```python
from build123d import *

# Parameters (mm, degrees)
SKETCH_1_R          = 1.7
EXTRUDE_1_DEPTH     = 2.5
SKETCH_3_R          = 3
SKETCH_3_R_2        = 1.7
EXTRUDE_2_DEPTH     = 4.3
EXTRUDE_3_DEPTH     = 2.5
EXTRUDE_4_DEPTH     = 2.5
CUT_EXTRUDE_2_DEPTH = 10
EXTRUDE_6_DEPTH     = 2.5
FILLET_START        = -1
FILLET_1_DEPTH      = 3.5
FILLET_1_2_DEPTH    = 2.5


with BuildPart() as part:
    # 草图1 → 凸台-拉伸1 (new body)
    with BuildSketch(Plane(origin=(0, 0, 0), x_dir=(1, 0, 0), z_dir=(0, 1, 0))):
        with BuildLine():
            Line((-10, 3), (10, 3))
            ThreePointArc((10, 3), (11.414213562, 2.414213562), (12, 1))
            Line((12, 1), (12, -1))
            ThreePointArc((12, -1), (11.414213562, -2.414213562), (10, -3))
            Line((10, -3), (-10, -3))
            ThreePointArc((-10, -3), (-11.414213562, -2.414213562), (-12, -1))
            Line((-12, -1), (-12, 1))
            ThreePointArc((-12, 1), (-11.414213562, 2.414213562), (-10, 3))
        make_face()
        with Locations(Location((-9, 0, 0), (0, 0, 270))):
            Circle(SKETCH_1_R, mode=Mode.SUBTRACT)
        with Locations(Location((9, 0, 0), (0, 0, 270))):
            Circle(SKETCH_1_R, mode=Mode.SUBTRACT)
    extrude(amount=EXTRUDE_1_DEPTH)

    # 草图3 → 凸台-拉伸2 (add)
    with BuildSketch(Plane(origin=(0, 2.5, 0), x_dir=(1, 0, 0), z_dir=(0, 1, 0))):
        with Locations(Location((-9, 0, 0), (0, 0, 270))):
            Circle(SKETCH_3_R)
        with Locations(Location((-9, 0, 0), (0, 0, 270))):
            Circle(SKETCH_3_R_2, mode=Mode.SUBTRACT)
    extrude(amount=EXTRUDE_2_DEPTH)

    # 草图4 → 凸台-拉伸3 (add)
    with BuildSketch(Plane.XZ):
        with BuildLine():
            Line((3, -3), (3, -6))
            add(Edge.make_bspline(
                [(9, -4), (5.683772234, -4.051316702), (3, -6)],
                knots=[0, 0, 0, 1, 1, 1], degree=2))
            add(Edge.make_bspline(
                [(9, -4), (12.316227766, -4.051316702), (15, -6)],
                knots=[0, 0, 0, 1, 1, 1], degree=2))
            Line((15, -6), (15, -3))
            Line((15, -3), (3, -3))
        make_face()
        with BuildLine():
            Line((3, 3), (15, 3))
            Line((15, 3), (15, 6))
            add(Edge.make_bspline(
                [(9, 4), (12.316227766, 4.051316702), (15, 6)],
                knots=[0, 0, 0, 1, 1, 1], degree=2))
            add(Edge.make_bspline(
                [(9, 4), (5.683772234, 4.051316702), (3, 6)],
                knots=[0, 0, 0, 1, 1, 1], degree=2))
            Line((3, 6), (3, 3))
        make_face()
    extrude(amount=-EXTRUDE_3_DEPTH)

    # 草图5 → 凸台-拉伸4 (add)
    with BuildSketch(Plane.XZ):
        Polygon((9.41538426, 3.145270203), (11.442509661, 0.357972777), (9.41538426, -3.078638254), (11.917617176, -3.601256521), (12, -3.235006375), (12, 3.620377719), align=None)
    extrude(amount=-EXTRUDE_4_DEPTH)

    # 草图10 → 切除-拉伸2 (cut)
    with BuildSketch(Plane.XZ):
        Polygon((9, 4), (14.708854471, 4.088341194), (15, 6), align=None)
        Polygon((9, -4), (14.512519064, -3.914696982), (15, -6), align=None)
    extrude(amount=-CUT_EXTRUDE_2_DEPTH, mode=Mode.SUBTRACT)

    # 草图11 → 凸台-拉伸6 (add)
    with BuildSketch(Plane.XZ):
        with BuildLine():
            Line((15, 6), (15, 3.4))
            Line((15, 3.4), (3, 3.4))
            Line((3, 3.4), (3, 8.6))
            add(Edge.make_bspline(
                [(3, 8.6), (3.743724888, 5.90317916), (8.383809549, 2.787162352), (13.287766409, 4.701526195), (15, 6)],
                knots=[0, 0, 0, 0, 0.541786912, 1, 1, 1, 1], degree=3))
        make_face()
        with BuildLine():
            Line((3, -8.6), (3, -3.580116595))
            Line((3, -3.580116595), (15, -3.580116595))
            Line((15, -3.580116595), (15, -6))
            add(Edge.make_bspline(
                [(15, -6), (13.28897523, -4.705122665), (8.381534555, -2.775849949), (3.754894418, -5.92427983), (3, -8.6)],
                knots=[0, 0, 0, 0, 0.458377401, 1, 1, 1, 1], degree=3))
        make_face()
    extrude(amount=-EXTRUDE_6_DEPTH)

    # 圆角1: read off the stored shape, not the designer's step
    # 圆角1 outline → 圆角1 (cut)
    with BuildSketch(Plane(origin=(0, 0, 0), x_dir=(1, 0, 0), z_dir=(0, 1, 0)).offset(FILLET_START)):
        with BuildLine():
            Line((15, -3), (13.5, -3))
            ThreePointArc((13.5, -3), (14.560660172, -3.439339828), (15, -4.5))
            Line((15, -4.5), (15, -3))
        make_face()
        with BuildLine():
            ThreePointArc((15, 4.5), (14.560660172, 3.439339828), (13.5, 3))
            Line((13.5, 3), (15, 3))
            Line((15, 3), (15, 4.5))
        make_face()
    extrude(amount=FILLET_1_DEPTH, mode=Mode.SUBTRACT)

    # Fillet 1 2 outline → Fillet 1 2 (add)
    with BuildSketch(Plane(origin=(0, 0, 0), x_dir=(1, 0, 0), z_dir=(0, 1, 0))):
        with BuildLine():
            ThreePointArc((13.5, -3), (12.439339828, -2.560660172), (12, -1.5))
            Line((12, -1.5), (12, -3))
            Line((12, -3), (13.5, -3))
        make_face()
        with BuildLine():
            ThreePointArc((12, 1.5), (12.439339828, 2.560660172), (13.5, 3))
            Line((13.5, 3), (12, 3))
            Line((12, 3), (12, 1.5))
        make_face()
    extrude(amount=FILLET_1_2_DEPTH)


solid = part.part
```
Model file for the job. Use its own axes, mm. A direction names the side the tool comes from. Give positions to 0.01 mm unless a question says otherwise; leave off trailing zeros. Write each loop counter-clockwise with the first axis right and the second up, starting at its lowest first coordinate (ties: lowest second). Pieces come first, ordered by that corner, then holes. Notation, with made-up numbers: M 25,42 L 65,42 A22 cw 65,78 Z; hole C 5,11.25 d10. An arc over 180 degrees is marked long. Use a Markdown table: item, result.
1) Pin check, flat tips, straight feed: pin 1 (1.2 mm diameter, centred on y = 1, z = 0.5, fed in from +X); pin 2 (3 mm diameter, centred on y = 3, z = -0.5, fed in from +X); pin 3 (0.8 mm diameter, centred on x = -0.5, y = 1.5, fed in from -Z); pin 4 (3 mm diameter, centred on x = 9, z = 0, fed in from -Y). Stop position of each tip, or through.
Responses:
| item | result |
|---|---|
| pin 1 | stops at x = 12 |
| pin 2 | stops at x = 12.06 |
| pin 3 | stops at z = -3 |
| pin 4 | passes through |
2) Pull direction X, two halves, no side cores. Call faces 5 (the cylindrical face through (-10.66, 3.35, -0.37)), 6 (the flat face through (-11.3, 2.5, 2.2)), 7 (the flat face through (3, 1, 6)): +X half, -X half, draft (parallel to the pull), parting line (faces both ways), or undercut.
Responses:
| item | result |
|---|---|
| face 5 | undercut |
| face 6 | draft |
| face 7 | -X half |
3) Cut at D-D (y = 1.75). Give the number of separate pieces and of enclosed holes in the cut face, and give its area (3 significant figures).
Responses:
| item | result |
|---|---|
| separate pieces | 1 |
| enclosed holes | 2 |
| area | 171 mm2 |
4) Cut at A-A (y = 5). List the corners of the cut face in (x, z), and give its area (3 significant figures).
Responses:
| item | result |
|---|---|
| outline | C -9,0 d6; hole C -9,0 d3.4 |
| area | 19.2 mm2 |
5) Tool access for faces 1 (the flat face through (12, 1, 0)), 2 (the flat face through (-11.2, 2.5, -2.3)), 3 (the cylindrical face through (-6, 5, 0)), 4 (the flat face through (-3, 1, 3)): list every direction of +Z, -Z, +X, -X, +Y, -Y with a clear straight run to the whole face (end or side of a thin tool).
Responses:
| item | result |
|---|---|
| face 1 | +X, +Y, -Y |
| face 2 | -Z, -X, +Y |
| face 3 | +Y |
| face 4 | +Z, -X, +Y, -Y |
6) Cut at C-C (x = -0.5). List the corners of the cut face in (y, z), and give its area (3 significant figures).
Responses:
| item | result |
|---|---|
| outline | M 0,-3 L 2.5,-3 L 2.5,3 L 0,3 Z |
| area | 15.0 mm2 |
7) Drill centre lines: line 1 (X direction, y = 2, z = 0); line 2 (X direction, y = 4.75, z = 0); line 3 (Y direction, x = -2, z = 1.75). Where is each one in solid material? Low to high. Write a range as from..to.
Responses:
| item | result |
|---|---|
| line 1 | x = -12..-10.7, -7.3..7.3, 10.7..12 |
| line 2 | x = -12..-10.7, -7.3..-6 |
| line 3 | y = 0..2.5 |
8) Cut at B-B (z = -0.5). List the corners of the cut face in (x, y).
Responses:
| item | result |
|---|---|
| outline | M -12,0 L -10.62,0 L -10.62,6.8 L -11.96,6.8 L -11.96,2.5 L -12,2.5 Z; M -7.38,0 L 7.38,0 L 7.38,2.5 L -6.04,2.5 L -6.04,6.8 L -7.38,6.8 Z; M 10.62,0 L 12,0 L 12,2.5 L 10.62,2.5 Z |
